Can you work these out from the model? Positions are in its coordinate system, mm. Coordinates: 2 decimals unless noted, no trailing zeros. Order: outer loops, then holes, each group sorted by start corner. A loop starts at its lowest first (then second) coordinate and runs counter-clockwise, first axis right, second up. Notation, with made-up numbers: (21.25, 11.25) - (33.25, 11.25) arc R19 ccw to (33.25, 31.25) - close; hole circle Ø10 at (51.25, -24.75). An arc over 180 degrees is marked (long way). Return JSON: item names as keys, results as strings. Group by question number.
1) If I drill on line 1 along Y through (x, z) = (-31.75, 1.85); line 2 along X through (y, z) = (-128.5, 1) (3 decimals); line 3 along Y through (x, z) = (-62.5, 2), over which ranges is the centre line in solid material (lowest first)?
2) If we mould it in two halves opening along X, with no side actions, what happens to faces 1 (the face through (-12, -17, 2.286)), 2 (the face through (48.924, 96.632, 1.127)), 3 (the face through (-87.2, -91.49, 1.13))? For each: pulls with the +X half, pulls with the -X half, needs draft (parallel to the pull), parting line crosses it, or undercut.
3) Imagine slicing it at A-A (z = 1.85). Give the number of separate pieces and of enclosed holes in the cut face, and give its area (3 significant figures).
4) Imagine slicing it at B-B (y = -149.5). Write out the boundary of the cut face in (x, z) (3 decimals).
5) Imagine slicing it at C-C (x = -70). Write out the boundary of the cut face in (y, z), and give its area (3 significant figures).
6) For pin 1 Ø2.5 at (x, y) = (-31.62, -112.54) entering from +Z; pin 2 Ø0.7 at (x, z) = (-64.5, 1.5) entering from -Y; pin 3 Ø1 at (x, z) = (33.5, 1) entering from +Y; pin 4 Ø1.1 at (y, z) = (-142, 1.5) entering from -X (3 decimals), each with a flat end and sliding along its axis, tell me the tip position at first contact or that it passes through.
```python
from build123d import *

# Parameters (mm, degrees)
BOSS_EXTRUDE1_DEPTH = 2.286
SKETCH18_R          = 1.5875
SKETCH18_R_2        = 1.016
CUT_EXTRUDE1_DEPTH  = 2.286


with BuildPart() as part:
    # Sketch1 → Boss-Extrude1 (new body)
    with BuildSketch(Plane.XY):
        Polygon((28.575, 108.380382361), (69.85, 84.55025), (69.85, -80.54975), (53.975, -102.122117639), (28.575, -102.122117639), (28.575, -171.972117639), (-53.975, -171.972117639), (-53.975, -102.122117639), (-79.375, -102.122117639), (-95.25, -80.54975), (-95.25, 84.55025), (-53.975, 108.380382361), (-53.975, 132.827882361), (28.575, 132.827882361), align=None)
    extrude(amount=BOSS_EXTRUDE1_DEPTH)

    # Sketch18 → Cut-Extrude1 (cut)
    with BuildSketch(Plane.XY.offset(2.286)):
        with Locations((-31.623, -159.272117639)):
            Circle(SKETCH18_R)
        with Locations((6.477, -159.272117639)):
            Circle(SKETCH18_R)
        with Locations((-31.75, 120.127882361)):
            Circle(SKETCH18_R)
        with Locations((6.35, 120.127882361)):
            Circle(SKETCH18_R)
        with Locations((-58.928, -83.072117639)):
            Circle(SKETCH18_R)
        with Locations((33.782, -83.072117639)):
            Circle(SKETCH18_R)
        with Locations((-58.928, 12.177882361)):
            Circle(SKETCH18_R)
        with Locations((33.782, 12.177882361)):
            Circle(SKETCH18_R)
        with Locations((-31.623, -112.536117639)):
            Circle(SKETCH18_R)
        with Locations((6.477, -112.536117639)):
            Circle(SKETCH18_R)
        with Locations((-49.784, 102.347882361)):
            Circle(SKETCH18_R_2)
        with Locations((24.384, 102.347882361)):
            Circle(SKETCH18_R_2)
        with Locations((-49.784, 19.162882361)):
            Circle(SKETCH18_R_2)
        with Locations((24.384, 19.162882361)):
            Circle(SKETCH18_R_2)
    extrude(amount=-CUT_EXTRUDE1_DEPTH, mode=Mode.SUBTRACT)


solid = part.part
```
Calculated:
{
 "1": {"line 1": "-171.97 to -160.85, -157.69 to -114.12, -110.95 to 118.54, 121.72 to 132.83", "line 2": "-53.975 to 28.575", "line 3": "-102.12 to 103.46"},
 "2": {"face 1": "needs draft", "face 2": "pulls with the +X half", "face 3": "pulls with the -X half"},
 "3": {"separate pieces": "1", "enclosed holes": "14", "area": "41,100 mm2"},
 "4": {"outline": "(-53.975, 0) - (28.575, 0) - (28.575, 2.286) - (-53.975, 2.286) - close"},
 "5": {"outline": "(-102.12, 0) - (99.13, 0) - (99.13, 2.29) - (-102.12, 2.29) - close", "area": "460 mm2"},
 "6": {"pin 1": "through", "pin 2": "y = -102.12", "pin 3": "y = 105.83", "pin 4": "x = -53.975"}
}
